Design review of the part shown in the three views and the two pictorial views. Dimensions are in mm from the part's minimum x, y and z. Round coordinates to 2 decimals unless told otherwise and drop trailing zeros. Loops run counter-clockwise (first coordinate to the right, second up) from the corner with the lowest first, then second, coordinate; pieces in that order, holes last. Notation, with made-up numbers: M -30,6 L -6,6 A21 ccw -6,30 Z; hole C 37,89 d2. An arc over 180 degrees is marked long. Answer as CSV lines item,"result". Start each with the question number.
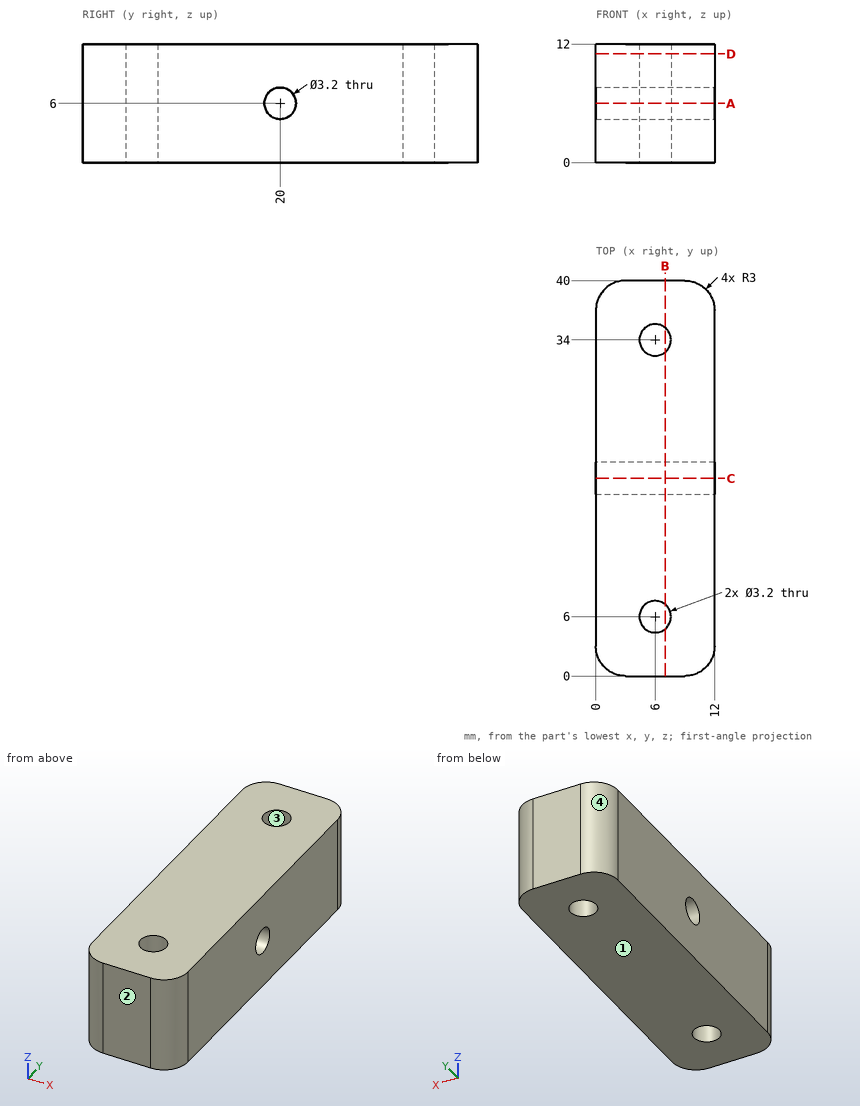
Item 1: Consider section D-D, the plane z = 11. Write out the cut boundary in (x, y).
Item 2: To check wall thickness, follow line 1 (Y direction, x = 4, z = 6); line 2 (Y direction, x = 6, z = 8.5); line 3 (Y direction, x = 6, z = 7). State the ranges of each line that lie inside material, in increasing order.
Item 3: The part is to be moulded in two halves that separate along Y. For the marked faces 1, 2, 3 and 4, say which applies: +Y half, -Y half, draft (parallel to the pull), parting line (faces both ways), or undercut.
Item 4: Consider section B-B, the plane x = 7. Write out the cut boundary in (y, z).
Item 5: Consider section A-A, the plane z = 6. Write out the cut boundary in (x, y).
Item 6: Insertion check: pin 1 Ø1.5 at (x, z) = (2, 5) entering from -Y; pin 2 Ø3 at (x, y) = (8, 15) entering from -Z; pin 3 Ø1.9 at (y, z) = (20, 6) entering from -X. Each pin has a flat end and moves straight along its axis. Give the tip position at first contact, or say it passes through.
Item 7: Consider section C-C, the plane y = 20. Write out the cut boundary in (x, z).
Found:
1,outline,"M 0,3 A3 ccw 3,0 L 9,0 A3 ccw 12,3 L 12,37 A3 ccw 9,40 L 3,40 A3 ccw 0,37 Z; hole C 6,6 d3.2; hole C 6,34 d3.2"
2,line 1,"y = 0 to 18.4, 21.6 to 40"
2,line 2,"y = 0 to 4.4, 7.6 to 32.4, 35.6 to 40"
2,line 3,"y = 0 to 4.4, 7.6 to 18.75, 21.25 to 32.4, 35.6 to 40"
3,face 1,"draft"
3,face 2,"-Y half"
3,face 3,"undercut"
3,face 4,"+Y half"
4,outline,"M 0,0 L 4.75,0 L 4.75,12 L 0,12 Z; M 7.25,0 L 32.75,0 L 32.75,12 L 7.25,12 Z; M 35.25,0 L 40,0 L 40,12 L 35.25,12 Z; hole C 20,6 d3.2"
5,outline,"M 0,3 A3 ccw 3,0 L 9,0 A3 ccw 12,3 L 12,18.4 L 0,18.4 Z; M 0,21.6 L 12,21.6 L 12,37 A3 ccw 9,40 L 3,40 A3 ccw 0,37 Z; hole C 6,6 d3.2; hole C 6,34 d3.2"
6,pin 1,"stops at y = 0.01"
6,pin 2,"stops at z = 0"
6,pin 3,"passes through"
7,outline,"M 0,0 L 12,0 L 12,4.4 L 0,4.4 Z; M 0,7.6 L 12,7.6 L 12,12 L 0,12 Z"
